Geometry check sheet. Reference: the model listing, model coordinates, mm. A direction names the side the tool comes from. Round coordinates to 2 decimals unless told otherwise and drop trailing zeros. Write each loop counter-clockwise with the first axis right and the second up, starting at its lowest first coordinate (ties: lowest second). Pieces come first, ordered by that corner, then holes. Notation, with made-up numbers: (6, 81) -> (50, 81) arc R18 cw to (50, 99) -> close; hole circle Ø2 at (79, 25). An arc over 180 degrees is marked (long way). Put each result on its own line as item: value. Start each with the question number.
from build123d import *

# Parameters (mm, degrees)
SKETCH1_W           = 220
SKETCH1_H           = 220
BOSS_EXTRUDE1_DEPTH = 300
SKETCH2_R           = 8
BOSS_EXTRUDE2_DEPTH = 80
FILLET1_R           = 20
FILLET2_R           = 5


with BuildPart() as part:
    # Sketch1 → Boss-Extrude1 (new body)
    with BuildSketch(Plane(origin=(0, 0, 0), x_dir=(1, 0, 0), z_dir=(0, 1, 0))):
        Rectangle(SKETCH1_W, SKETCH1_H)
    extrude(amount=BOSS_EXTRUDE1_DEPTH)

    # Sketch2 → Boss-Extrude2 (add)
    with BuildSketch(Plane(origin=(0, 300, 0), x_dir=(1, 0, 0), z_dir=(0, 1, 0))):
        with Locations(Location((0, 0, 0), (0, 0, 90))):
            Circle(SKETCH2_R)
    extrude(amount=BOSS_EXTRUDE2_DEPTH)

    # Fillet1
    fillet1_edges = [part.edges().sort_by_distance(p)[0] for p in [
        (-110, 150, -110),
        (110, 150, -110),
        (110, 150, 110),
        (-110, 150, 110),
    ]]
    fillet(fillet1_edges, radius=FILLET1_R)

    # Fillet2
    fillet2_edges = [part.edges().sort_by_distance(p)[0] for p in [
        (0, 380, 8),
    ]]
    fillet(fillet2_edges, radius=FILLET2_R)


solid = part.part
(1) Material ranges on L1, parallel to Y at x = -34.5, z = -90; L2, parallel to Z at x = 91, y = 124.5; L3, parallel to X at y = 29.5, z = -99, recorded low to high. Write a range as from..to.
(2) Sectioned sample at C-C (y = 326). Record the cut outline in (x, z).
(3) Sectioned sample at B-B (z = 27). Record the cut outline in (x, y), and give its area (3 significant figures).
(4) Sectioned sample at A-A (x = -25.5). Record the cut outline in (y, z), and give its area (3 significant figures).
(5) Go/stop test with a flat-tipped pin: pin 1 Ø1.5 at (x, z) = (67.5, 86) entering from +Y. Record where the tip stops, or that it passes through.
(6) Set-up check for faces 1 (the cylindrical face through (-104.297, 152.1, -103.986)), 2 (the cylindrical face through (7.81, 336.98, 1.73)): record each of +Z, -Z, +X, -X, +Y, -Y from which the full face is reachable in a straight line by a thin tool's end or side.
Found:
1. L1: 0..300
1. L2: -109.97..109.97
1. L3: -107.86..107.86
2. outline: circle Ø16 at (0, 0)
3. outline: (-110, 0) -> (110, 0) -> (110, 300) -> (-110, 300) -> close
3. area: 66,000 mm2
4. outline: (0, -110) -> (300, -110) -> (300, 110) -> (0, 110) -> close
4. area: 66,000 mm2
5. pin 1: y = 300
6. face 1: -Z, -X, +Y, -Y
6. face 2: +Y
